Job drawing, mm, ordinate dimensions from the low corner. One solid piece. A direction names the side the tool comes from. Round coordinates to 2 decimals unless told otherwise and drop trailing zeros. Loops run counter-clockwise (first coordinate to the right, second up) from the corner with the lowest first, then second, coordinate; pieces in that order, holes last.
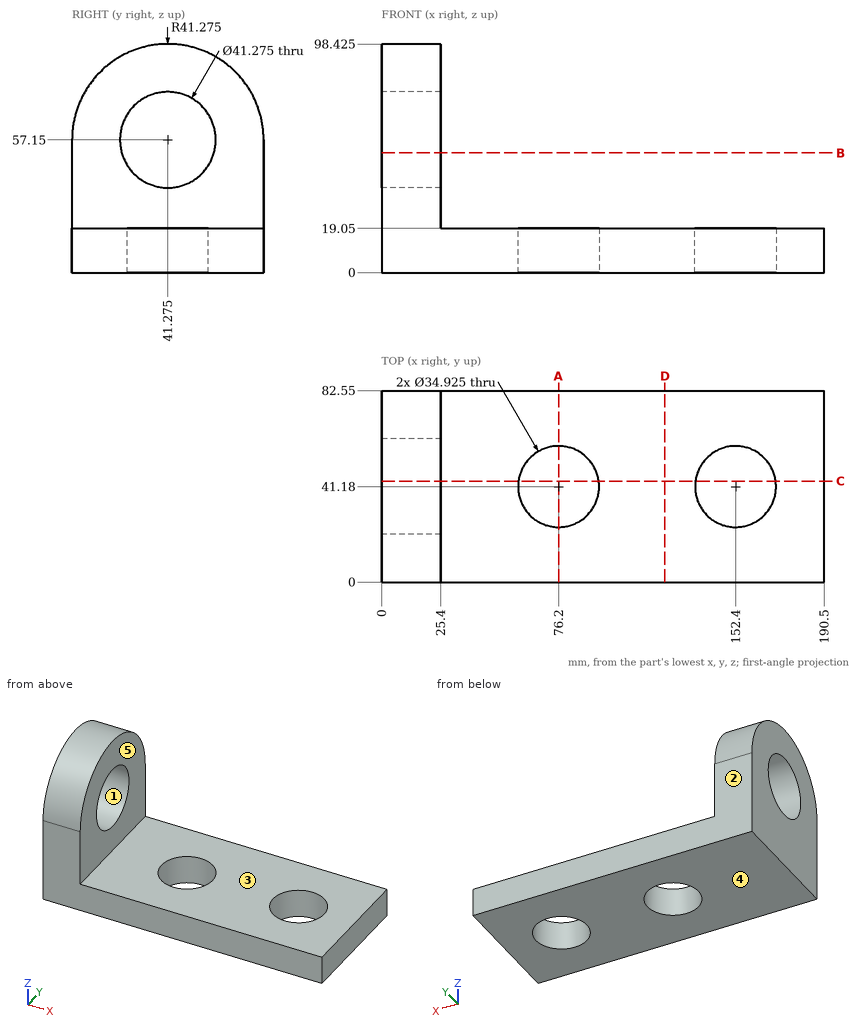
Item 1: Flat gauge pins, fed straight in: P1, Ø5, axis at x = 57, y = 63.5, coming from the +Z side; P2, Ø6, axis at x = 20, y = 37.5, coming from the +Z side; P3, Ø12, axis at y = 69.5, z = 72.5, coming from the +X side. Where does each tip first touch, or does it go through?
Answers follow:
P1: stops at z = 19.05
P2: stops at z = 98.42
P3: stops at x = 25.4
Item 2: Two-plate mould, pull along Y, no slides. Class the marked faces 1, 2 and 3: released by +Y, released by -Y, zero draft, split by the parting line, or undercut.
Answers follow:
face 1: undercut
face 2: released by +Y
face 3: zero draft
Item 3: Cut at C-C, the plane y = 43.5. Give the cut face in (x, z) (3 decimals), plus the area to 3 significant figures.
Answers follow:
outline: (0, 0) - (58.892, 0) - (58.892, 19.05) - (25.4, 19.05) - (25.4, 36.633) - (0, 36.633) - close; (0, 77.667) - (25.4, 77.667) - (25.4, 98.365) - (0, 98.365) - close; (93.508, 0) - (135.092, 0) - (135.092, 19.05) - (93.508, 19.05) - close; (169.708, 0) - (190.5, 0) - (190.5, 19.05) - (169.708, 19.05) - close
area: 3,280 mm2
Item 4: Cut at B-B, the plane z = 51.5. Give the cut face in (x, y).
Answers follow:
outline: (0, 0) - (25.4, 0) - (25.4, 21.43) - (0, 21.43) - close; (0, 61.12) - (25.4, 61.12) - (25.4, 82.55) - (0, 82.55) - close
Item 5: Cut at D-D, the plane x = 122. Give the cut face in (y, z), plus the area to 3 significant figures.
Answers follow:
outline: (0, 0) - (82.55, 0) - (82.55, 19.05) - (0, 19.05) - close
area: 1,570 mm2
Item 6: 3-axis set-ups, long thin cutter, end or side, ignore diameter. For the marked faces 4 and 5: which of +Z, -Z, +X, -X, +Y, -Y reach the whole face in a straight line?
Answers follow:
face 4: -Z, +X, -X, +Y, -Y
face 5: +Z, +X, +Y, -Y
Item 7: Probe line 1 (X direction, y = 40, z = 16); line 2 (Y direction, x = 6, z = 57); line 3 (Y direction, x = 152, z = 10). List the from-to ranges inside material, lowest first.
Answers follow:
line 1: x = 0 to 58.78, 93.62 to 134.98, 169.82 to 190.5
line 2: y = 0 to 20.64, 61.91 to 82.55
line 3: y = 0 to 23.72, 58.64 to 82.55
Item 8: Cut at A-A, the plane x = 76.2. Give the cut face in (y, z), plus the area to 3 significant figures.
Answers follow:
outline: (0, 0) - (23.72, 0) - (23.72, 19.05) - (0, 19.05) - close; (58.64, 0) - (82.55, 0) - (82.55, 19.05) - (58.64, 19.05) - close
area: 907 mm2
